from build123d import *

# Parameters (mm, degrees)
F0_W     = 152.4
F0_H     = 152.4
F1_DEPTH = 152.4
F2_W     = 114.3
F2_H     = 114.3
F3_DEPTH = 152.4
F4_R     = 38.1
F5_DEPTH = 76.2
F7_DEPTH = 304.8


with BuildPart() as f1:
    # F0 (on Front) → F1 (new body)
    with BuildSketch(Plane.XZ):
        with Locations((76.2, 76.2)):
            Rectangle(F0_W, F0_H)
    extrude(amount=F1_DEPTH)

    # F2 (on face) → F3 (cut)
    with BuildSketch(Plane.XZ.offset(152.4)):
        with Locations((95.25, 95.25)):
            Rectangle(F2_W, F2_H)
    extrude(amount=-F3_DEPTH, mode=Mode.SUBTRACT)

    # F4 (on face) → F5 (cut)
    with BuildSketch(Plane.XY.offset(38.1)):
        with Locations((152.4, -76.2)):
            Circle(F4_R)
    extrude(amount=-F5_DEPTH, mode=Mode.SUBTRACT)

    # F6 (on face) → F7 (cut)
    with BuildSketch(Plane.YZ.offset(38.1)):
        with BuildLine():
            Line((-76.2, 152.4), (-152.4, 152.4))
            Line((-152.4, 152.4), (-152.4, 76.2))
            ThreePointArc((-152.4, 76.2), (-130.081537, 130.081537), (-76.2, 152.4))
        make_face()
        with BuildLine():
            Line((0, 152.4), (-76.2, 152.4))
            ThreePointArc((-76.2, 152.4), (-22.318463, 130.081537), (0, 76.2))
            Line((0, 76.2), (0, 152.4))
        make_face()
    extrude(amount=-F7_DEPTH, mode=Mode.SUBTRACT)


solid = f1.part
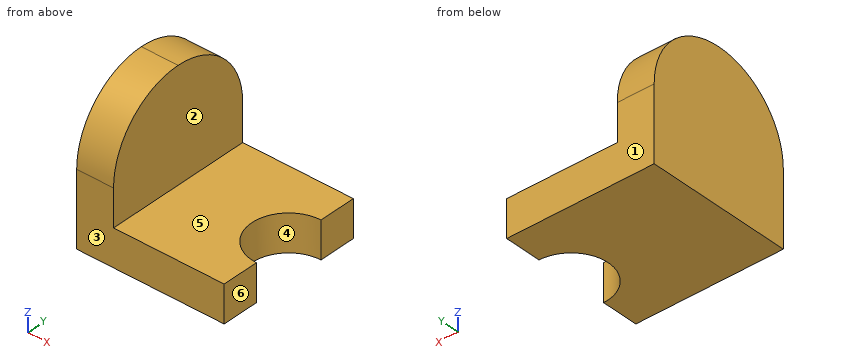
Work out the finished part from the listing and answer in its coordinate system (mm). Face numbers are marked on the shaded views. A direction names the side the tool comes from. Give positions to 0.01 mm unless a question says otherwise; leave off trailing zeros. Order: outer loops, then holes, each group sorted by start corner. A loop starts at its lowest first (then second) coordinate and runs counter-clockwise, first axis right, second up. Notation, with made-up numbers: M 8.5,77 L 41.5,77 A12 ccw 41.5,89 Z; hole C -35,71.5 d7. An arc over 180 degrees is marked long. Return JSON: item names as keys, results as strings.
Q1. Find the intervals of material crossed by line 1 along Z through (x, y) = (133.5, -145); line 2 along Z through (x, y) = (35, -23.5), in increasing order. Write a range as [from, to].
Answer below:
{"line 1": "z = [0, 38.1]", "line 2": "z = [0, 131.24]"}
Q2. Find section B-B, the plane x = 33.5. Write down the section's boundary in (y, z), and give its area (3 significant figures).
Answer below:
{"outline": "M -152.4,0 L 0,0 L 0,76.2 A76.2 ccw -76.2,152.4 A76.2 ccw -152.4,76.2 Z", "area": "20,700 mm^2"}
Q3. Each of these flat-tipped pins is pushed along its axis until it touches: pin 1 (8 mm diameter, centred on x = 79, y = -62, fed in from +Z); pin 2 (2 mm diameter, centred on y = -86.5, z = 135, fed in from +X). Where does it stop, or does it pass through?
Answer below:
{"pin 1": "stops at z = 38.1", "pin 2": "stops at x = 38.1"}
Q4. Find section D-D, the plane y = -124. Write down the section's boundary in (x, z), and give its area (3 significant figures).
Answer below:
{"outline": "M 0,0 L 152.4,0 L 152.4,38.1 L 38.1,38.1 L 38.1,135.54 L 0,135.54 Z", "area": "9,520 mm^2"}
Q5. The mould has two halves that part along Y. Classify the marked faces 1, 2, 3 and 4: pulls with the +Y half, pulls with the -Y half, needs draft (parallel to the pull), parting line crosses it, or undercut.
Answer below:
{"face 1": "pulls with the +Y half", "face 2": "needs draft", "face 3": "pulls with the -Y half", "face 4": "undercut"}
Q6. Find section A-A, the plane x = 122.5. Write down the section's boundary in (y, z).
Answer below:
{"outline": "M -152.4,0 L -99.81,0 L -99.81,38.1 L -152.4,38.1 Z; M -52.59,0 L 0,0 L 0,38.1 L -52.59,38.1 Z"}
Q7. Which of the six approach directions +Z, -Z, +X, -X, +Y, -Y give full straight-line access (tool end or side, diameter ignored) to the marked faces 5 and 6?
Answer below:
{"face 5": "+Z, +X, +Y, -Y", "face 6": "+Z, -Z, +X, +Y, -Y"}
Q8. Find section C-C, the plane z = 34. Write down the section's boundary in (x, y).
Answer below:
{"outline": "M 0,-152.4 L 152.4,-152.4 L 152.4,-114.3 A38.1 cw 152.4,-38.1 L 152.4,0 L 0,0 Z"}
